```python
from build123d import *

# Parameters (mm, degrees)
CROQUIS1_R            = 15
CROQUIS1_R_2          = 10
EXTRUIR_L_MINA1_DEPTH = 2.5
CROQUIS2_R            = 12.5
CROQUIS2_R_2          = 10
EXTRUIR_L_MINA2_DEPTH = 45
REDONDEO3_R           = 1
CROQUIS5_R            = 12.5
CROQUIS5_R_2          = 10
EXTRUIR_L_MINA3_DEPTH = 25
CROQUIS6_R            = 15
CROQUIS6_R_2          = 10
EXTRUIR_L_MINA4_DEPTH = 2.5
REDONDEO4_R           = 1
CROQUIS7_R            = 10
CORTAR_EXTRUIR1_DEPTH = 51
CROQUIS8_R            = 10
CORTAR_EXTRUIR2_DEPTH = 28


with BuildPart() as part:
    # Croquis1 → Extruir-Lámina1 (new body)
    with BuildSketch(Plane.XY):
        Circle(CROQUIS1_R)
        Circle(CROQUIS1_R_2, mode=Mode.SUBTRACT)
    extruir_l_mina1 = extrude(amount=EXTRUIR_L_MINA1_DEPTH)

    # Croquis2 → Extruir-Lámina2 (add)
    with BuildSketch(Plane(origin=(0, 0, 0), x_dir=(-1, 0, 0), z_dir=(0, 0, -1))):
        Circle(CROQUIS2_R)
        Circle(CROQUIS2_R_2, mode=Mode.SUBTRACT)
    extrude(amount=EXTRUIR_L_MINA2_DEPTH)

    # Simetría1: Extruir-Lámina1 across plane
    add(extruir_l_mina1.mirror(Plane.XY.offset(-22.5)))

    # Redondeo3
    redondeo3_edges = [part.edges().sort_by_distance(p)[0] for p in [
        (-15, 0, -45),
        (-15, 0, 0),
    ]]
    fillet(redondeo3_edges, radius=REDONDEO3_R)

    # Croquis5 → Extruir-Lámina3 (add)
    with BuildSketch(Plane(origin=(0, 0, 0), x_dir=(1, 0, 0), z_dir=(0, 1, 0))):
        with Locations((0, 22.5)):
            Circle(CROQUIS5_R)
        with Locations((0, 22.5)):
            Circle(CROQUIS5_R_2, mode=Mode.SUBTRACT)
    extrude(amount=EXTRUIR_L_MINA3_DEPTH)

    # Croquis6 → Extruir-Lámina4 (add)
    with BuildSketch(Plane(origin=(0, 25, 0), x_dir=(1, 0, 0), z_dir=(0, 1, 0))):
        with Locations((0, 22.5)):
            Circle(CROQUIS6_R)
        with Locations((0, 22.5)):
            Circle(CROQUIS6_R_2, mode=Mode.SUBTRACT)
    extrude(amount=EXTRUIR_L_MINA4_DEPTH)

    # Redondeo4
    redondeo4_edges = [part.edges().sort_by_distance(p)[0] for p in [
        (-15, 25, -22.5),
    ]]
    fillet(redondeo4_edges, radius=REDONDEO4_R)

    # Croquis7 → Cortar-Extruir1 (cut, through all)
    with BuildSketch(Plane(origin=(0, 0, -47.5), x_dir=(-1, 0, 0), z_dir=(0, 0, -1))):
        Circle(CROQUIS7_R)
    extrude(amount=-CORTAR_EXTRUIR1_DEPTH, mode=Mode.SUBTRACT)

    # Croquis8 → Cortar-Extruir2 (cut)
    with BuildSketch(Plane(origin=(0, 27.5, 0), x_dir=(1, 0, 0), z_dir=(0, 1, 0))):
        with Locations((0, 22.5)):
            Circle(CROQUIS8_R)
    extrude(amount=-CORTAR_EXTRUIR2_DEPTH, mode=Mode.SUBTRACT)


solid = part.part
```
The model under review builds one solid part; all positions refer to its coordinate system, in mm. A direction names the side the tool comes from. Round coordinates to 2 decimals unless told otherwise and drop trailing zeros. Loops run counter-clockwise (first coordinate to the right, second up) from the corner with the lowest first, then second, coordinate; pieces in that order, holes last. Notation, with made-up numbers: M 81,-25 L 129,-25 A16 ccw 129,-7 Z; hole C 30.25,-37 d9. An arc over 180 degrees is marked long. Put each result on its own line as item: value.
Q1. Consider section C-C, the plane x = -5.75. Count the separate pieces of the cut face and the enclosed holes in it, then the cut area to 3 significant figures.
Result set:
separate pieces: 3
enclosed holes: 0
area: 380 mm²
Q2. For pin 1 (6 mm diameter, centred on x = 3, z = -21.5, fed in from +Y); pin 2 (4 mm diameter, centred on x = -10, z = -8, fed in from -Y); pin 3 (6 mm diameter, centred on x = -8, y = 21.5, fed in from -Z), all flat-tipped, find the tip position at first contact; note any pin that passes through.
Result set:
pin 1: stops at y = -8
pin 2: stops at y = -9.6
pin 3: stops at z = -33.96
Q3. Machinability: for faces 4 (the flat face through (-5.3, 11.5, -45)), 5 (the cylindrical face through (-3.252, 26.74, -7.857)), 6 (the cylindrical face through (-14.985, 0.66, 1.74)), which of the approach directions +Z, -Z, +X, -X, +Y, -Y give a long, thin tool a straight path to every point of the face, cutting with its end or side? Answer none if there is none.
Result set:
face 4: none
face 5: +Y
face 6: +Z
Q4. To check wall thickness, follow L1, parallel to X at y = 18, z = -22.5; L2, parallel to Z at x = 0, y = 20.5; L3, parallel to X at y = 15, z = -20. State the ranges of each line that lie inside material, in increasing order.
Result set:
L1: x = -12.5 to -10, 10 to 12.5
L2: z = -35 to -32.5, -12.5 to -10
L3: x = -12.25 to -9.68, 9.68 to 12.25
Q5. Consider section A-A, the plane z = -1.5. Give the boundary of the cut face in (x, y).
Result set:
outline: C 0,0 d25; hole C 0,0 d20
Q6. Mouldability with a two-part tool opening along Z and no side actions: class faces 1 (the cylindrical face through (2.71, -12.203, -22.185)), 2 (the flat face through (3, -10, 2.5)), 3 (the flat face through (3.1, 27.5, -12.7)) as released by +Z, released by -Z, zero draft, split by the parting line, or undercut.
Result set:
face 1: undercut
face 2: released by +Z
face 3: zero draft
Q7. Consider section B-B, the plane y = 21. Give the boundary of the cut face in (x, z), then the cut area to 3 significant figures.
Result set:
outline: C 0,-22.5 d25; hole C 0,-22.5 d20
area: 177 mm²
